Could you check a few things on this model? Use its own coordinates, in mm. A direction names the side the tool comes from. Give positions to 0.01 mm unless a question says otherwise; leave off trailing zeros. Order: outer loops, then holes, each group sorted by start corner. A loop starts at its lowest first (then second) coordinate and runs counter-clockwise, first axis right, second up.
(1) Imagine slicing it at C-C, the plane x = -40.75. Write out the boundary of the cut face in (y, z), then the cut area to 4 significant figures.
(2) If we mould it in two halves opening along X, with no side actions, what happens to faces 4 (the flat face through (-32, 5, 38)), 5 (the flat face through (-27.844, 2, 42)), 6 (the flat face through (-36, 1, 35.366))? For each: released by +X, released by -X, zero draft, split by the parting line, or undercut.
(3) Imagine slicing it at A-A, the plane y = 0.5. Write out the boundary of the cut face in (x, z).
(4) Will this pin go through, and if not, where does the flat tip stop? pin 1 (5 mm diameter, centred on x = -39, z = 38.5, fed in from -Y).
(5) Imagine slicing it at B-B, the plane z = 42.5. Write out the boundary of the cut face in (x, y).
(6) If I drill on probe 1 along Z at (x, y) = (-41, 1.75); probe 2 along X at (y, z) = (1.05, 35.5); probe 3 along Y at (x, z) = (-29.5, 40.5), over which ranges is the centre line in solid material (lowest first)?
(7) On a 3-axis mill with a long thin cutter (end or side, diameter ignored), from which of +Z, -Z, +X, -X, +Y, -Y can I reach the whole of each face in a straight line? I mean faces 1 (the flat face through (-36, 2, 33.866)), 2 (the cylindrical face through (-30.871, 4.037, 35.555)), 3 (the flat face through (-36, 1.9, 42)). Say none if no direction works.
(8) Imagine slicing it at D-D, the plane y = 4.15. Write out the boundary of the cut face in (x, z) (3 decimals), then the cut area to 3 significant figures.
from build123d import *

# Parameters (mm, degrees)
SKETCH1_W           = 15.9
SKETCH1_H           = 15.9
BOSS_EXTRUDE1_DEPTH = 3.1
SKETCH2_W           = 12.9
SKETCH2_H           = 12.9
CUT_EXTRUDE1_DEPTH  = 1.9
SKETCH3_R           = 2.475
BOSS_EXTRUDE2_DEPTH = 1.9


with BuildPart() as part:
    # Sketch1 → Boss-Extrude1 (new body)
    with BuildSketch(Plane(origin=(0, 0, 0), x_dir=(1, 0, 0), z_dir=(0, 1, 0))):
        with Locations((-35.79416664, -41.816451592)):
            Rectangle(SKETCH1_W, SKETCH1_H)
    extrude(amount=BOSS_EXTRUDE1_DEPTH)

    # Sketch2 → Cut-Extrude1 (cut)
    with BuildSketch(Plane.XZ):
        with Locations((-35.79416664, 41.816451592)):
            Rectangle(SKETCH2_W, SKETCH2_H)
    extrude(amount=-CUT_EXTRUDE1_DEPTH, mode=Mode.SUBTRACT)

    # Sketch3 → Boss-Extrude2 (add)
    with BuildSketch(Plane(origin=(0, 3.1, 0), x_dir=(1, 0, 0), z_dir=(0, 1, 0))):
        with Locations(Location((-39.76916664, -37.841451592, 0), (0, 0, 90))):
            Circle(SKETCH3_R)
        with Locations(Location((-31.81916664, -37.841451592, 0), (0, 0, 90))):
            Circle(SKETCH3_R)
        with Locations(Location((-39.76916664, -45.791451592, 0), (0, 0, 90))):
            Circle(SKETCH3_R)
        with Locations(Location((-31.81916664, -45.791451592, 0), (0, 0, 90))):
            Circle(SKETCH3_R)
    extrude(amount=BOSS_EXTRUDE2_DEPTH)


solid = part.part
Answer block:
1. outline: (0, 33.87) - (3.1, 33.87) - (3.1, 35.57) - (5, 35.57) - (5, 40.11) - (3.1, 40.11) - (3.1, 43.52) - (5, 43.52) - (5, 48.06) - (3.1, 48.06) - (3.1, 49.77) - (0, 49.77) - (0, 48.27) - (1.9, 48.27) - (1.9, 35.37) - (0, 35.37) - close
1. area: 42.05 mm2
2. face 4: zero draft
2. face 5: released by +X
2. face 6: undercut
3. outline: (-43.74, 33.87) - (-27.84, 33.87) - (-27.84, 49.77) - (-43.74, 49.77) - close; hole (-42.24, 35.37) - (-29.34, 35.37) - (-29.34, 48.27) - (-42.24, 48.27) - close
4. pin 1: stops at y = 1.9
5. outline: (-43.74, 0) - (-42.24, 0) - (-42.24, 1.9) - (-29.34, 1.9) - (-29.34, 0) - (-27.84, 0) - (-27.84, 3.1) - (-43.74, 3.1) - close
6. probe 1: z = 33.87 to 35.37, 48.27 to 49.77
6. probe 2: x = -43.74 to -42.24, -29.34 to -27.84
6. probe 3: y = 1.9 to 3.1
7. face 1: -Z, +X, -X, +Y, -Y
7. face 2: +Y
7. face 3: -Y
8. outline: circle Ø4.95 at (-39.769, 37.841); circle Ø4.95 at (-39.769, 45.791); circle Ø4.95 at (-31.819, 37.841); circle Ø4.95 at (-31.819, 45.791)
8. area: 77.0 mm2
